Source: CAD feature listing. Evaluate the final solid. Frame: model axes, mm. Face numbers are marked on the shaded views. A direction names the side the tool comes from. Round coordinates to 2 decimals unless told otherwise and drop trailing zeros. Loops run counter-clockwise (first coordinate to the right, second up) from the corner with the lowest first, then second, coordinate; pieces in that order, holes last. Notation, with made-up numbers: (-25, 51.5) - (-2, 51.5) arc R19 cw to (-2, 73.5) - close; hole circle Ø10 at (7.5, 29). An arc over 180 degrees is marked (long way). One line per question, with ' | ' between items. Start each with the question number.
1. Cut plane D-D (z = 22.5). Return loops of the section in (x, y), then the cut area to 3 significant figures.
2. Cut plane C-C (x = 106). Return loops of the section in (y, z).
3. Mould query, pull axis Z, two halves, no side actions, for the marked faces 1, 2, 3 and 4. Classes: pulls with the +Z half, pulls with the -Z half, needs draft (parallel to the pull), parting line crosses it, or undercut.
4. Pin query (flat end, axial travel): pin 1 (1.8 mm diameter, centred on y = -85, z = 27, fed in from +X); pin 2 (0.7 mm diameter, centred on x = 85, y = -86.5, fed in from +Z); pin 3 (3 mm diameter, centred on y = -86, z = 24, fed in from -X); pin 4 (3 mm diameter, centred on x = 102.22, z = -2, fed in from -Y) (3 decimals). Return the tip coordinate at first contact, or that it passes through.
5. Cut plane A-A (z = 14.5). Return loops of the section in (x, y).
6. Cut plane B-B (z = -2). Return loops of the section in (x, y).
7. Access query for the marked faces 5, 6, 7, 8 and 9. Directions: +Z, -Z, +X, -X, +Y, -Y. A direction counts if a zero-diameter tool reaches every point of the face in a straight line with its end or side. Return the directions, or none.
8. Ray query, line 1 (X direction, y = -83.05, z = 16); line 2 (X direction, y = -83.5, z = -2); line 3 (Z direction, x = 80.5, y = -87.45). Return the intervals inside material, ascending.
```python
from build123d import *

# Parameters (mm, degrees)
DODANIE_WYCI_GNI_CIE1_DEPTH      = 20
DODANIE_WYCI_GNI_CIE1_DEPTH_BACK = 6
SZKIC1_W                         = 35
SZKIC1_H                         = 6
WYTNIJ_WYCI_GNI_CIE1_DEPTH       = 112.693205508
SZKIC4_R                         = 1.55
WYTNIJ_WYCI_GNI_CIE2_DEPTH       = 6
SZKIC6_W                         = 11
SZKIC6_H                         = 6
DODANIE_WYCI_GNI_CIE2_DEPTH      = 10
SZYK_LINIOWY1_COUNT              = 2
SZYK_LINIOWY1_PITCH              = 19
WYTNIJ_WYCI_GNI_CIE3_DEPTH       = 6


with BuildPart() as part:
    # Szkic1 → Dodanie-wyciągnięcie1 (new, two sides: drawn at the far end of the back side and taken through both)
    with BuildSketch(Plane.XY.offset(-DODANIE_WYCI_GNI_CIE1_DEPTH_BACK)):
        with Locations((92.224072822, -85.062373271)):
            Rectangle(SZKIC1_W, SZKIC1_H)
    extrude(amount=DODANIE_WYCI_GNI_CIE1_DEPTH + DODANIE_WYCI_GNI_CIE1_DEPTH_BACK)

    # Szkic3 → Wytnij-wyciągnięcie1 (cut, through all)
    with BuildSketch(Plane.XZ.offset(88.062373271)):
        Polygon((103.274072822, 20), (100.174072822, 20), (100.174072822, 12), (98.799072822, 12), (98.799072822, 10), (100.174072822, 10), (100.174072822, 9.5), (103.274072822, 9.5), (103.274072822, 10), (104.649072822, 10), (104.649072822, 12), (103.274072822, 12), align=None)
    wytnij_wyci_gni_cie1 = extrude(amount=-WYTNIJ_WYCI_GNI_CIE1_DEPTH, mode=Mode.SUBTRACT)

    # Szkic4 → Wytnij-wyciągnięcie2 (cut)
    with BuildSketch(Plane.XZ.offset(88.062373271)):
        with Locations(Location((102.224072822, -2, 0), (0, 0, 270))):
            Circle(SZKIC4_R)
    extrude(amount=-WYTNIJ_WYCI_GNI_CIE2_DEPTH, mode=Mode.SUBTRACT)

    # Szkic6 → Dodanie-wyciągnięcie2 (add)
    with BuildSketch(Plane.XY.offset(20)):
        with Locations((92.224072822, -85.062373271)):
            Rectangle(SZKIC6_W, SZKIC6_H)
    extrude(amount=DODANIE_WYCI_GNI_CIE2_DEPTH)

    # Szyk liniowy1: Wytnij-wyciągnięcie1 ×2
    with Locations(*[(-i * SZYK_LINIOWY1_PITCH, 0, 0) for i in range(1, SZYK_LINIOWY1_COUNT)]):
        add(wytnij_wyci_gni_cie1, mode=Mode.SUBTRACT)

    # Szkic7 → Wytnij-wyciągnięcie3 (cut)
    with BuildSketch(Plane.XZ.offset(88.062373271)):
        with BuildLine():
            Line((109.724072822, -4), (109.724072822, -6))
            Line((109.724072822, -6), (107.724072822, -6))
            ThreePointArc((107.724072822, -6), (109.138286384, -5.414213562), (109.724072822, -4))
        make_face()
        with BuildLine():
            Line((76.724072822, -6), (74.724072822, -6))
            Line((74.724072822, -6), (74.724072822, -4))
            ThreePointArc((74.724072822, -4), (75.30985926, -5.414213562), (76.724072822, -6))
        make_face()
    extrude(amount=-WYTNIJ_WYCI_GNI_CIE3_DEPTH, mode=Mode.SUBTRACT)


solid = part.part
```
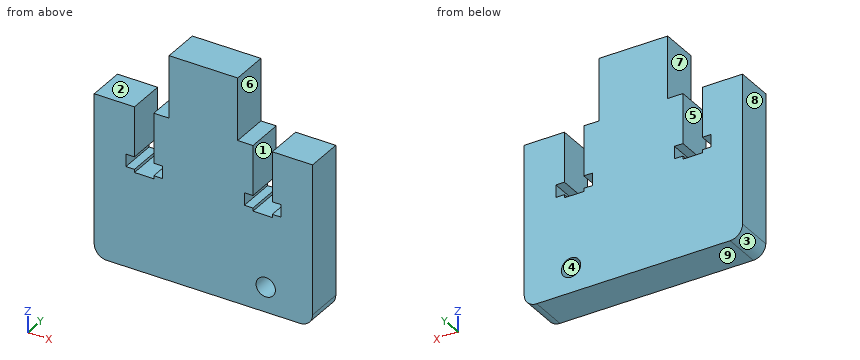
Answers follow:
1) outline: (86.72, -88.06) - (97.72, -88.06) - (97.72, -82.06) - (86.72, -82.06) - close | area: 66.0 mm2
2) outline: (-88.06, -6) - (-82.06, -6) - (-82.06, 20) - (-88.06, 20) - close
3) face 1: needs draft | face 2: pulls with the +Z half | face 3: pulls with the -Z half | face 4: undercut
4) pin 1: stops at x = 97.72 | pin 2: stops at z = 20 | pin 3: stops at x = 86.72 | pin 4: passes through
5) outline: (74.72, -88.06) - (81.17, -88.06) - (81.17, -82.06) - (74.72, -82.06) - close; (84.27, -88.06) - (100.17, -88.06) - (100.17, -82.06) - (84.27, -82.06) - close; (103.27, -88.06) - (109.72, -88.06) - (109.72, -82.06) - (103.27, -82.06) - close
6) outline: (74.72, -88.06) - (100.67, -88.06) - (100.67, -82.06) - (74.72, -82.06) - close; (103.77, -88.06) - (109.72, -88.06) - (109.72, -82.06) - (103.77, -82.06) - close
7) face 5: +Z, +Y, -Y | face 6: +Z, +X, +Y, -Y | face 7: +Z, -X, +Y, -Y | face 8: +Z, -Z, -X, +Y, -Y | face 9: -Z, +X, -X, +Y, -Y
8) line 1: x = 74.72 to 81.17, 84.27 to 100.17, 103.27 to 109.72 | line 2: x = 74.72 to 100.67, 103.77 to 109.72 | line 3: z = -6 to 10, 12 to 20
